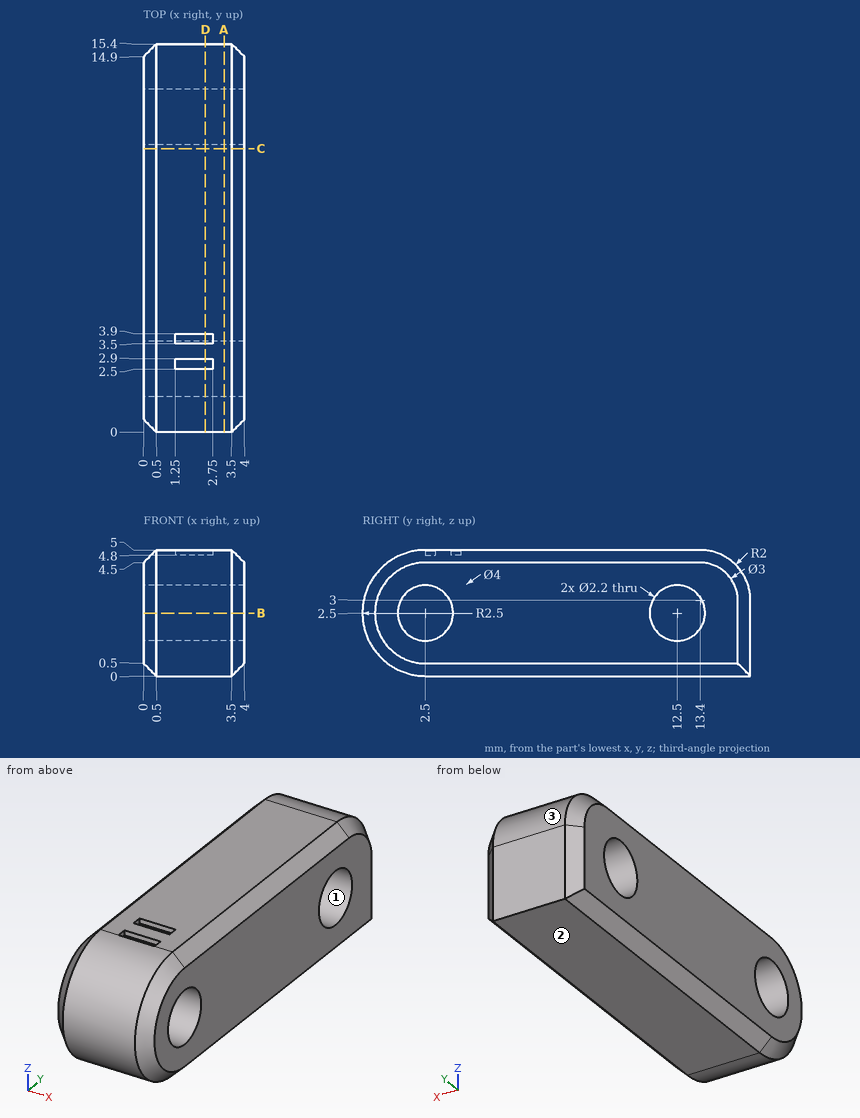
Geometry check sheet. Reference: drawing and pictorial views, mm from the part's lowest x, y, z. Give positions to 0.01 mm unless a question says otherwise; leave off trailing zeros. Loops run counter-clockwise (first coordinate to the right, second up) from the corner with the lowest first, then second, coordinate; pieces in that order, holes last. Notation, with made-up numbers: (49, 35) -> (69, 35) arc R34 cw to (69, 71) -> close; hole circle Ø5 at (-9, -12.75). An arc over 180 degrees is marked (long way). Answer in a Markdown table with one row per item. Add a question column.
1) Cross-section at C-C on y = 11.25. Record the boundary of the cut face in (x, z).
2) Material ranges on probe 1 along Z at (x, y) = (2.8, 12.5); probe 2 along Y at (x, z) = (0.85, 2.3); probe 3 along Y at (x, z) = (0.2, 2.7), recorded low to high. Write a range as from..to.
3) Draft check along Z on the marked faces 1, 2 and 3. Enter one of: pulls with the +Z half, pulls with the -Z half, needs draft (parallel to the pull), parting line crosses it, or undercut.
4) Cross-section at A-A on x = 3.2. Record the boundary of the cut face in (y, z), and give its area (3 significant figures).
5) Cross-section at B-B on z = 2.5. Record the boundary of the cut face in (x, y).
6) Cross-section at D-D on x = 2.45. Record the boundary of the cut face in (y, z).
Outcome:
| question | item | result |
|---|---|---|
| 1 | outline | (0, 0.5) -> (0.5, 0) -> (3.5, 0) -> (4, 0.5) -> (4, 4.5) -> (3.5, 5) -> (0.5, 5) -> (0, 4.5) -> close |
| 2 | probe 1 | z = 0..1.4, 3.6..5 |
| 2 | probe 2 | y = 0.01..1.42, 3.58..11.42, 13.58..15.4 |
| 2 | probe 3 | y = 0.31..1.42, 3.58..11.42, 13.58..15.1 |
| 3 | face 1 | undercut |
| 3 | face 2 | pulls with the -Z half |
| 3 | face 3 | pulls with the +Z half |
| 4 | outline | (2.5, 0) -> (15.4, 0) -> (15.4, 3) arc R2 ccw to (13.4, 5) -> (2.5, 5) arc R2.5 ccw to start; hole circle Ø2.2 at (2.5, 2.5); hole circle Ø2.2 at (12.5, 2.5) |
| 4 | area | 65.9 mm^2 |
| 5 | outline | (0, 0.5) -> (0.5, 0) -> (3.5, 0) -> (4, 0.5) -> (4, 1.4) -> (0, 1.4) -> close; (0, 3.6) -> (4, 3.6) -> (4, 11.4) -> (0, 11.4) -> close; (0, 13.6) -> (4, 13.6) -> (4, 14.9) -> (3.5, 15.4) -> (0.5, 15.4) -> (0, 14.9) -> close |
| 6 | outline | (2.5, 0) -> (15.4, 0) -> (15.4, 3) arc R2 ccw to (13.4, 5) -> (3.9, 5) -> (3.9, 4.8) -> (3.5, 4.8) -> (3.5, 5) -> (2.9, 5) -> (2.9, 4.8) -> (2.5, 4.8) -> (2.5, 5) arc R2.5 ccw to start; hole circle Ø2.2 at (2.5, 2.5); hole circle Ø2.2 at (12.5, 2.5) |
